```python
from build123d import *

# Parameters (mm, degrees)
F1_DEPTH    = 12.7
F2_R        = 2.54
F3_T1_DEPTH = 40.1963065702
F4_R        = 2.54


# Not quite as in the source:
# - a fillet or chamfer that OpenCascade refuses, or shapes differently, is made with other operations: its cross-section is extruded or revolved along the edge and cut away or added


with BuildPart() as f1:
    # F0 (on Top) → F1 (new body)
    with BuildSketch(Plane.XY):
        with BuildLine():
            Line((0, 5.08), (0, -5.08))
            Line((0, -5.08), (3.175, -5.08))
            Line((3.175, -5.08), (3.175, 1.905))
            ThreePointArc((3.175, 1.905), (5.1435, 3.8735), (7.112, 1.905))
            Line((7.112, 1.905), (7.112, 0))
            Line((7.112, 0), (9.017, 0))
            Line((9.017, 0), (9.017, 5.08))
            Line((9.017, 5.08), (0, 5.08))
        make_face()
    extrude(amount=F1_DEPTH)

    # F2
    f2_edges = [f1.edges().sort_by_distance(p)[0] for p in [
        (9.017, 5.08, 6.35),
    ]]
    fillet(f2_edges, radius=F2_R)

    # F3: fillet of radius 6.35 on 1 edges, made by hand

    # F3_s2 → F3_t1 (cut)
    with BuildSketch(Plane.XY.offset(-13.7481532851)):
        with BuildLine():
            ThreePointArc((0, -5.08), (2.324261314, -2.755738686), (3.175, 0.419261314))
            Line((3.175, 0.419261314), (3.175, -5.08))
            Line((3.175, -5.08), (0, -5.08))
        make_face()
    extrude(amount=F3_T1_DEPTH, mode=Mode.SUBTRACT)

    # F4
    f4_edges = [f1.edges().sort_by_distance(p)[0] for p in [
        (8.0645, 0, 12.7),
        (8.0645, 0, 0),
    ]]
    fillet(f4_edges, radius=F4_R)


solid = f1.part
```
Geometry check sheet. Reference: the model listing, model coordinates, mm. A direction names the side the tool comes from. Coordinates: 2 decimals unless noted, no trailing zeros. Order: outer loops, then holes, each group sorted by start corner. A loop starts at its lowest first (then second) coordinate and runs counter-clockwise, first axis right, second up. Notation, with made-up numbers: (86, 78) - (123, 78) arc R11 ccw to (123, 92) - close; hole circle Ø10 at (18, 67). An arc over 180 degrees is marked (long way). Answer in a Markdown table with one row per item. Add a question column.
1. Gauge pin test, flat ends, axial feed: pin 1 Ø0.6 at (x, z) = (8.5, 5) entering from -Y; pin 2 Ø5 at (x, y) = (6.5, -1) entering from +Z; pin 3 Ø1.5 at (y, z) = (-1, 8.5) entering from +X. Record the tip position at first contact, or that the pin passes through.
2. Section check A-A (y = 1.75). Enter the section's corners in (x, z) (3 decimals), plus the area to 3 significant figures.
3. Access from +Z, -Z, +X, -X, +Y, -Y to the whole of each face (thin tool, end or side, straight path). Record for faces 5 (the face through (8.026, 0.724, 11.936)), 6 (the face through (8.026, 0.764, 0.724)), 7 (the face through (3.175, 1, 6)).
4. Material ranges on L1, parallel to X at y = 0.5, z = 9 (3 decimals); L2, parallel to X at y = -3, z = 9.5; L3, parallel to Y at x = 0.5, z = 0.75, recorded low to high. Write a range as [from, to].
5. Section check D-D (y = -2.5). Enter the section's corners in (x, z), plus the area to 3 significant figures.
6. Draft check along X on faces 1 (the face through (8.29, 4.32, 6.44)), 2 (the face through (7.112, 1, 6)), 3 (the face through (8, 0, 6)), 4 (the face through (0, 0, 6)). Enter one of: +X half, -X half, draft (parallel to the pull), parting line (faces both ways), or undercut.
7. Section check C-C (y = 0.25). Enter the section's corners in (x, z), plus the area to 3 significant figures.
Data:
| question | item | result |
|---|---|---|
| 1 | pin 1 | stops at y = 0 |
| 1 | pin 2 | stops at z = 12.44 |
| 1 | pin 3 | stops at x = 3.14 |
| 2 | outline | (0, 0) - (3.175, 0) - (3.175, 12.7) - (0, 12.7) - close; (7.112, 0.126) - (9.017, 0.126) - (9.017, 12.574) - (7.112, 12.574) - close |
| 2 | area | 64.0 mm² |
| 3 | face 5 | +Z, +X, -Y |
| 3 | face 6 | -Z, +X, -Y |
| 3 | face 7 | +Z, -Z, -Y |
| 4 | L1 | x = [0, 3.175], [7.112, 9.017] |
| 4 | L2 | x = [0, 2.18] |
| 4 | L3 | y = [-4.76, 5.08] |
| 5 | outline | (0, 0) - (2.46, 0) - (2.46, 12.7) - (0, 12.7) - close |
| 5 | area | 31.3 mm² |
| 6 | face 1 | +X half |
| 6 | face 2 | undercut |
| 6 | face 3 | draft |
| 6 | face 4 | -X half |
| 7 | outline | (0, 0) - (3.17, 0) - (3.17, 12.7) - (0, 12.7) - close; (7.11, 1.44) - (9.02, 1.44) - (9.02, 11.26) - (7.11, 11.26) - close |
| 7 | area | 59.0 mm² |
